Input: part model. Units: mm. Frame: model coordinates. Face numbers are marked on the shaded views. A direction names the side the tool comes from. Coordinates: 2 decimals unless noted, no trailing zeros. Loops run counter-clockwise (first coordinate to the right, second up) from the corner with the lowest first, then second, coordinate; pieces in that order, holes last. Notation, with made-up numbers: M -34.5,14 L 22.5,14 A31 cw 22.5,39 Z; hole C 72,81.5 d10. An arc over 180 degrees is marked long. Use a Markdown table: item, result. Add a question column.
1. Line query: L1, parallel to X at y = 0.5, z = -12.1; L2, parallel to X at y = 2.5, z = -12.1; L3, parallel to Z at x = -3.75, y = 4.25. Output: solid intervals per line, ascending. Write a range as [from, to].
2. Section D-D on x = -8. Output: boundary loops of the cut face in (y, z), then the cut area to 3 significant figures.
3. Draft query along X for the marked faces 1, 2 and 3. Return one class per face: +X half, -X half, draft (parallel to the pull), parting line (faces both ways), or undercut.
4. Section A-A on z = 12.1. Output: boundary loops of the cut face in (x, y), then the cut area to 3 significant figures.
5. Section C-C on y = 9. Output: boundary loops of the cut face in (x, z).
6. Set-up query: the marked faces 4, 5 and 6. Return all of +Z, -Z, +X, -X, +Y, -Y with unobstructed straight access to the full face (end or side cutting, diameter ignored); none if empty.
7. Pin query (flat end, axial travel): pin 1 (1 mm diameter, centred on x = 4.5, y = 9, fed in from +Z); pin 2 (6.5 mm diameter, centred on x = 8.5, z = -13.5, fed in from +Y); pin 3 (8 mm diameter, centred on x = 10, z = 2.5, fed in from +Y); pin 4 (4 mm diameter, centred on x = -10, y = 7, fed in from -Z). Return the tip coordinate at first contact, or that it passes through.
8. Section B-B on x = 0. State how many separate pieces and enclosed holes the cut face has, then the cut area to 3 significant figures.
```python
from build123d import *

# Parameters (mm, degrees)
EXTRUDE_1_DEPTH           = 4
SKETCH_2_R                = 1.5
CUT_EXTRUDE_2_DEPTH       = 23.365375025
SKETCH_3_R                = 3
CUT_EXTRUDE_3_DEPTH       = 3
FILLET_1_R                = 3
SKETCH_4_W                = 15
SKETCH_4_H                = 12
EXTRUDE_2_DEPTH           = 10
CUT_EXTRUDE_7_DEPTH       = 31.229786635
SKETCH_9_R                = 2.75
EXTRUDE_3_DEPTH           = 3
SKETCH_10_R               = 1.5
CUT_EXTRUDE_8_DEPTH       = 28.20680062
CUT_EXTRUDE_9_REACH       = 29.207
CUT_EXTRUDE_9_END_RADIUS  = 122
CUT_EXTRUDE_13_REACH      = 29.207
CUT_EXTRUDE_13_END_RADIUS = 119
SKETCH_12_W               = 8
SKETCH_12_H               = 6


with BuildPart() as part:
    # 草图1 → 凸台-拉伸1 (new body)
    with BuildSketch(Plane(origin=(0, 0, 0), x_dir=(1, 0, 0), z_dir=(0, 1, 0))):
        Polygon((-15, 16.1), (-4.1, 16.1), (-4.1, 8.1), (4.1, 8.1), (4.1, 16.1), (15, 16.1), (15, -8.1), (3.9, -8.1), (3.9, -16.1), (-3.9, -16.1), (-3.9, -8.1), (-15, -8.1), align=None)
    extrude(amount=EXTRUDE_1_DEPTH)

    # 草图2 → 切除-拉伸2 (cut, through all)
    with BuildSketch(Plane(origin=(0, 0, 0), x_dir=(1, 0, 0), z_dir=(0, 1, 0))):
        with Locations(Location((-8, 12.1, 0), (0, 0, 270))):
            Circle(SKETCH_2_R)
        with Locations(Location((8, 12.1, 0), (0, 0, 270))):
            Circle(SKETCH_2_R)
        with Locations(Location((0, -12.1, 0), (0, 0, 270))):
            Circle(SKETCH_2_R)
    extrude(amount=CUT_EXTRUDE_2_DEPTH, mode=Mode.SUBTRACT)

    # 草图3 → 切除-拉伸3 (cut)
    with BuildSketch(Plane(origin=(0, 4, 0), x_dir=(1, 0, 0), z_dir=(0, 1, 0))):
        with Locations(Location((-8, 12.1, 0), (0, 0, 270))):
            Circle(SKETCH_3_R)
        with Locations(Location((8, 12.1, 0), (0, 0, 270))):
            Circle(SKETCH_3_R)
        with Locations(Location((0, -12.1, 0), (0, 0, 270))):
            Circle(SKETCH_3_R)
    extrude(amount=-CUT_EXTRUDE_3_DEPTH, mode=Mode.SUBTRACT)

    # 圆角1
    fillet_1_edges = [part.edges().sort_by_distance(p)[0] for p in [
        (-15, 2, -16.1),
        (-4.1, 2, -16.1),
        (4.1, 2, -16.1),
        (15, 2, -16.1),
        (15, 2, 8.1),
        (3.9, 2, 16.1),
        (-3.9, 2, 16.1),
        (-15, 2, 8.1),
    ]]
    fillet(fillet_1_edges, radius=FILLET_1_R)

    # 草图4 → 凸台-拉伸2 (add)
    with BuildSketch(Plane(origin=(0, 4, 0), x_dir=(1, 0, 0), z_dir=(0, 1, 0))):
        with Locations((0, 0.1)):
            Rectangle(SKETCH_4_W, SKETCH_4_H)
    extrude(amount=EXTRUDE_2_DEPTH)

    # 草图8 → 切除-拉伸7 (cut, through all)
    with BuildSketch(Plane(origin=(0, 0, -6.1), x_dir=(-1, 0, 0), z_dir=(0, 0, -1))):
        with BuildLine():
            Line((-7.5, 13), (-7.5, 14))
            Line((-7.5, 14), (7.5, 14))
            Line((7.5, 14), (7.5, 13))
            ThreePointArc((7.5, 13), (0, 13.225202865), (-7.5, 13))
        make_face()
    extrude(amount=-CUT_EXTRUDE_7_DEPTH, mode=Mode.SUBTRACT)

    # 草图9 → 凸台-拉伸3 (add)
    with BuildSketch(Plane(origin=(0, 13, 0), x_dir=(-1, 0, 0), z_dir=(0, -1, 0))):
        with Locations(Location((0, 0.1, 0), (0, 0, 180))):
            Circle(SKETCH_9_R)
    extrude(amount=-EXTRUDE_3_DEPTH)

    # 草图10 → 切除-拉伸8 (cut, through all)
    with BuildSketch(Plane(origin=(0, 16, 0), x_dir=(1, 0, 0), z_dir=(0, 1, 0))):
        with Locations(Location((0, 0, 0), (0, 0, 180))):
            Circle(SKETCH_10_R)
    extrude(amount=-CUT_EXTRUDE_8_DEPTH, mode=Mode.SUBTRACT)

    # 切除-拉伸9: up to this cylinder (the profile starts inside it)
    cut_extrude_9_end = Plane(origin=(0, -111.774797135, 0), z_dir=(0, 0, -1)) * Cylinder(CUT_EXTRUDE_9_END_RADIUS, 303.414, mode=Mode.PRIVATE)
    # 草图11 → 切除-拉伸9 (cut, up to the surface)
    with BuildSketch(Plane.XZ, mode=Mode.PRIVATE) as cut_extrude_9_sk1:
        Polygon((3.175426481, 0), (1.58771324, 2.75), (-1.58771324, 2.75), (-3.175426481, 0), (-1.58771324, -2.75), (1.58771324, -2.75), align=None)
    cut_extrude_9_tool1 = extrude(cut_extrude_9_sk1.sketch, amount=-CUT_EXTRUDE_9_REACH, mode=Mode.PRIVATE) & cut_extrude_9_end
    add(cut_extrude_9_tool1.solids().sort_by_distance((0, 0, 0))[0], mode=Mode.SUBTRACT)

    # 切除-拉伸13: up to this cylinder (the profile starts inside it)
    cut_extrude_13_end = Plane(origin=(0, -111.774797135, 0), z_dir=(0, 0, -1)) * Cylinder(CUT_EXTRUDE_13_END_RADIUS, 297.414, mode=Mode.PRIVATE)
    # 草图12 → 切除-拉伸13 (cut, up to the surface)
    with BuildSketch(Plane.XZ, mode=Mode.PRIVATE) as cut_extrude_13_sk1:
        Rectangle(SKETCH_12_W, SKETCH_12_H)
    cut_extrude_13_tool1 = extrude(cut_extrude_13_sk1.sketch, amount=-CUT_EXTRUDE_13_REACH, mode=Mode.PRIVATE) & cut_extrude_13_end
    add(cut_extrude_13_tool1.solids().sort_by_distance((0, 0, 0))[0], mode=Mode.SUBTRACT)


solid = part.part
```
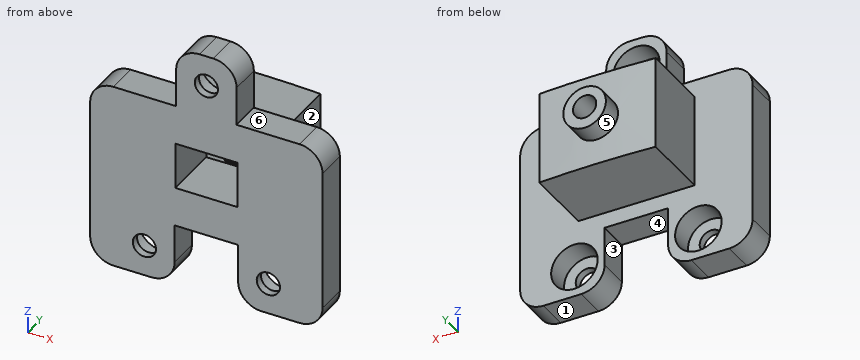
Answers below:
| question | item | result |
|---|---|---|
| 1 | L1 | x = [-15, -9.5], [-6.5, -4.1], [4.1, 6.5], [9.5, 15] |
| 1 | L2 | x = [-15, -11], [-5, -4.1], [4.1, 5], [11, 15] |
| 1 | L3 | z = [-6.1, -3], [3, 5.9] |
| 2 | outline | M 0,-16.1 L 4,-16.1 L 4,-15.1 L 1,-15.1 L 1,-13.6 L 0,-13.6 Z; M 0,-10.6 L 1,-10.6 L 1,-9.1 L 4,-9.1 L 4,8.1 L 0,8.1 Z |
| 2 | area | 75.8 mm² |
| 3 | face 1 | draft |
| 3 | face 2 | +X half |
| 3 | face 3 | undercut |
| 4 | outline | M -3.9,0 L -1.5,0 L -1.5,1 L -3,1 L -3,4 L -3.9,4 Z; M 1.5,0 L 3.9,0 L 3.9,4 L 3,4 L 3,1 L 1.5,1 Z |
| 4 | area | 10.2 mm² |
| 5 | outline | M -7.5,-6.1 L 7.5,-6.1 L 7.5,5.9 L -7.5,5.9 Z; hole M -3.18,0 L -1.59,-2.75 L 1.59,-2.75 L 3.18,0 L 1.59,2.75 L -1.59,2.75 Z |
| 6 | face 4 | -Z, +Y, -Y |
| 6 | face 5 | +Y |
| 6 | face 6 | +Z, +X, +Y, -Y |
| 7 | pin 1 | stops at z = 5.9 |
| 7 | pin 2 | stops at y = 4 |
| 7 | pin 3 | stops at y = 13.08 |
| 7 | pin 4 | passes through |
| 8 | separate pieces | 3 |
| 8 | enclosed holes | 0 |
| 8 | area | 125 mm² |
